Can you work these out from the model? Positions are in its coordinate system, mm. A direction names the side the tool comes from. Round coordinates to 2 decimals unless told otherwise and drop trailing zeros. Loops run counter-clockwise (first coordinate to the right, second up) from the corner with the lowest first, then second, coordinate; pieces in that order, holes last. Notation, with made-up numbers: (7, 27.5) -> (41, 27.5) arc R19 cw to (41, 42.5) -> close; hole circle Ø10 at (20, 76). An arc over 180 degrees is marked (long way). Answer as a JSON object with one key per item and string values.
```python
from build123d import *

# Parameters (mm, degrees)
F0_W        = 7
F0_H        = 10
F1_DEPTH    = 25
F2_R        = 10
F3_DEPTH    = 5
F4_T        = 2.5
F4_T3_DEPTH = 30


# Not quite as in the source:
# - a shell that OpenCascade refuses in one call is made with other operations: the cavity is built on its own and cut out


with BuildPart() as f1:
    # F0 (on Right) → F1 (new body)
    with BuildSketch(Plane.YZ):
        with Locations((-3.5, 30)):
            Rectangle(F0_W, F0_H)
        Polygon((-32, 0), (0, 0), (0, 25), (-7, 25), (-32, 25), align=None)
    extrude(amount=F1_DEPTH)

    # F2 (on face) → F3 (cut)
    with BuildSketch(Plane.XY.offset(25)):
        with Locations((12.5, -19.5)):
            Circle(F2_R)
    extrude(amount=-F3_DEPTH, mode=Mode.SUBTRACT)

    # F4: shell of thickness 2.5, made by hand


with BuildPart() as f4_core1:
    # F4_t2: copy of F1
    add(f1.part)

    # the walls: a layer under each face that stays
    f4_faces = [f4_core1.faces().sort_by_distance(p)[0] for p in [
        (12.5, -3.5, 35),
        (12.5, 0, 17.5),
        (12.5, -7, 30),
        (0, -16, 17.5),
        (25, -16, 17.5),
        (20.8333333333, -11.1666666667, 25),
        (12.5, -32, 12.5),
        (2.5, -19.5, 22.5),
        (12.5, -19.5, 20),
    ]]
    thicken(f4_faces, amount=-F4_T, mode=Mode.SUBTRACT)

    # F4_s4 → F4_t3 (cut)
    with BuildSketch(Plane.YZ.offset(-2.5)):
        Polygon((-7.025, 25.025), (-4.5, 25), (-4.5, 22.5), (-7, 22.5), align=None)
    extrude(amount=F4_T3_DEPTH, mode=Mode.SUBTRACT)

    # F4_s5 → F4_t6 (revolve, cut)
    with BuildSketch(Plane.XZ.offset(19.5)):
        Polygon((22.475, 20.025), (25, 20), (25, 17.5), (22.5, 17.5), align=None)
    revolve(axis=Axis((12.5, -19.5, 20), (0, 0, 1)), mode=Mode.SUBTRACT)


with BuildPart() as f1_1:
    add(f1.part)

    # what is left inside the walls is the cavity
    f4_cavity = [f4_core1.part.solids().sort_by_distance(p)[0] for p in [
        (15.833333, -2.525, 16.25),
    ]]
    add(f4_cavity, mode=Mode.SUBTRACT)


solid = f1_1.part
```
Q1. We'd pull the mould along Y, two halves only. Please class faces 1 (the cylindrical face through (12.7, -7, 20)), 2 (the flat face through (12, 0, 17)), 3 (the flat face through (12, -7, 30)), 4 (the flat face through (25, -16, 14)): pulls with the +Y half, pulls with the -Y half, needs draft (parallel to the pull), parting line crosses it, or undercut.
Determined:
{"face 1": "undercut", "face 2": "pulls with the +Y half", "face 3": "pulls with the -Y half", "face 4": "needs draft"}
Q2. I want a section at C-C, the plane y = -19.5. Write out the boundary of the cut face in (x, z), then the cut area to 3 significant figures.
Determined:
{"outline": "(0, 0) -> (2.5, 0) -> (2.5, 17.5) -> (22.5, 17.5) -> (22.5, 0) -> (25, 0) -> (25, 25) -> (22.5, 25) -> (22.5, 20) -> (2.5, 20) -> (2.5, 25) -> (0, 25) -> close", "area": "175 mm²"}
Q3. If I drill on L1, parallel to Y at x = 12.5, z = 21.4; L2, parallel to Y at x = 12.5, z = 22.8; L3, parallel to X at y = -5.5, z = 2, over which ranges is the centre line in solid material (lowest first)? Write a range as [from, to].
Determined:
{"L1": "[-32, -29.5], [-9.5, -7], [-2.5, 0]", "L2": "[-32, -29.5], [-9.5, -4.5], [-2.5, 0]", "L3": "[0, 2.5], [22.5, 25]"}
Q4. I want a section at B-B, the plane z = 23. Write out the boundary of the cut face in (x, y), then the cut area to 3 significant figures.
Determined:
{"outline": "(0, -32) -> (25, -32) -> (25, 0) -> (0, 0) -> close; hole circle Ø20 at (12.5, -19.5); hole (2.5, -4.5) -> (22.5, -4.5) -> (22.5, -2.5) -> (2.5, -2.5) -> close", "area": "446 mm²"}
Q5. I want a section at D-D, the plane x = 12.5. Write out the boundary of the cut face in (y, z), then the cut area to 3 significant figures.
Determined:
{"outline": "(-32, 0) -> (-29.5, 0) -> (-29.5, 17.5) -> (-7, 17.5) -> (-7, 22.5) -> (-4.5, 22.5) -> (-4.5, 32.5) -> (-2.5, 32.5) -> (-2.5, 0) -> (0, 0) -> (0, 35) -> (-7, 35) -> (-7, 25) -> (-9.5, 25) -> (-9.5, 20) -> (-29.5, 20) -> (-29.5, 25) -> (-32, 25) -> close", "area": "255 mm²"}
Q6. I'm going to push flat-ended pins straight in: pin 1 (12 mm diameter, centred on x = 12.5, y = -19.5, fed in from -Z); pin 2 (1 mm diameter, centred on y = -14.5, z = 27, fed in from +X); pin 3 (1 mm diameter, centred on x = 16.5, y = -17.5, fed in from +Z); pin 4 (0.6 mm diameter, centred on x = 13, y = -3.5, fed in from -Z). Where does each tip first touch, or does it pass through?
Determined:
{"pin 1": "z = 17.5", "pin 2": "through", "pin 3": "z = 20", "pin 4": "z = 32.5"}
Q7. I want a section at A-A, the plane z = 26.5. Write out the boundary of the cut face in (x, y).
Determined:
{"outline": "(0, -7) -> (25, -7) -> (25, 0) -> (0, 0) -> close; hole (2.5, -4.5) -> (22.5, -4.5) -> (22.5, -2.5) -> (2.5, -2.5) -> close"}
Q8. On a 3-axis mill with a long thin cutter (end or side, diameter ignored), from which of +Z, -Z, +X, -X, +Y, -Y can I reach the whole of each face in a straight line? I mean faces 5 (the flat face through (23, -16, 0)), 6 (the flat face through (12, -4.5, 27)), 7 (the flat face through (12, -19, 20)). Say none if no direction works.
Determined:
{"face 5": "-Z, +X, -X, +Y, -Y", "face 6": "-Z", "face 7": "+Z"}
